```python
from build123d import *

# Parameters (mm, degrees)
SKETCH3_W           = 50.8
SKETCH3_H           = 25.4
SKETCH3_W_2         = 45.72
SKETCH3_H_2         = 20.32
BOSS_EXTRUDE1_DEPTH = 711.2
SKETCH5_R           = 5.08
CUT_EXTRUDE2_DEPTH  = 127


with BuildPart() as part:
    # Sketch3 → Boss-Extrude1 (new body)
    with BuildSketch(Plane(origin=(0, 0, 0), x_dir=(0, 0, -1), z_dir=(1, 0, 0))):
        with Locations((5.321216632, -1.999606833)):
            Rectangle(SKETCH3_W, SKETCH3_H)
        with Locations((5.321216632, -1.999606833)):
            Rectangle(SKETCH3_W_2, SKETCH3_H_2, mode=Mode.SUBTRACT)
    extrude(amount=BOSS_EXTRUDE1_DEPTH)

    # Sketch5 → Cut-Extrude2 (cut)
    with BuildSketch(Plane.XY.offset(20.078783368)):
        with Locations((10.978833808, -1.999606833)):
            Circle(SKETCH5_R)
        with Locations((36.378833808, -1.999606833)):
            Circle(SKETCH5_R)
        with Locations((61.778833808, -1.999606833)):
            Circle(SKETCH5_R)
        with Locations((87.178833808, -1.999606833)):
            Circle(SKETCH5_R)
        with Locations((112.578833808, -1.999606833)):
            Circle(SKETCH5_R)
        with Locations((137.978833808, -1.999606833)):
            Circle(SKETCH5_R)
        with Locations((163.378833808, -1.999606833)):
            Circle(SKETCH5_R)
        with Locations((188.778833808, -1.999606833)):
            Circle(SKETCH5_R)
        with Locations((214.178833808, -1.999606833)):
            Circle(SKETCH5_R)
        with Locations((239.578833808, -1.999606833)):
            Circle(SKETCH5_R)
        with Locations((264.978833808, -1.999606833)):
            Circle(SKETCH5_R)
        with Locations((290.378833808, -1.999606833)):
            Circle(SKETCH5_R)
        with Locations((315.778833808, -1.999606833)):
            Circle(SKETCH5_R)
        with Locations((341.178833808, -1.999606833)):
            Circle(SKETCH5_R)
        with Locations((366.578833808, -1.999606833)):
            Circle(SKETCH5_R)
        with Locations((391.978833808, -1.999606833)):
            Circle(SKETCH5_R)
        with Locations((417.378833808, -1.999606833)):
            Circle(SKETCH5_R)
        with Locations((442.778833808, -1.999606833)):
            Circle(SKETCH5_R)
        with Locations((468.178833808, -1.999606833)):
            Circle(SKETCH5_R)
        with Locations((493.578833808, -1.999606833)):
            Circle(SKETCH5_R)
        with Locations((518.978833808, -1.999606833)):
            Circle(SKETCH5_R)
        with Locations((544.378833808, -1.999606833)):
            Circle(SKETCH5_R)
        with Locations((569.778833808, -1.999606833)):
            Circle(SKETCH5_R)
        with Locations((595.178833808, -1.999606833)):
            Circle(SKETCH5_R)
        with Locations((620.578833808, -1.999606833)):
            Circle(SKETCH5_R)
        with Locations((645.978833808, -1.999606833)):
            Circle(SKETCH5_R)
        with Locations((671.378833808, -1.999606833)):
            Circle(SKETCH5_R)
        with Locations((696.778833808, -1.999606833)):
            Circle(SKETCH5_R)
    extrude(amount=-CUT_EXTRUDE2_DEPTH, mode=Mode.SUBTRACT)


solid = part.part
```
The listing builds one solid part. Answer for the finished solid, in the listing's coordinates (mm). A direction names the side the tool comes from. Give positions to 0.01 mm unless a question says otherwise; leave off trailing zeros. Order: outer loops, then holes, each group sorted by start corner. A loop starts at its lowest first (then second) coordinate and runs counter-clockwise, first axis right, second up.
1) Find section A-A on z = 2.5. Write down the section's boundary in (x, y), then the cut area to 3 significant figures.
Reported:
outline: (0, -14.7) - (711.2, -14.7) - (711.2, -12.16) - (0, -12.16) - close; (0, 8.16) - (711.2, 8.16) - (711.2, 10.7) - (0, 10.7) - close
area: 3,610 mm2
2) Consider line 1 along Z through (x, y) = (43.5, 2.75); line 2 along Y through (x, z) = (214, 4.5); line 3 along Y through (x, z) = (235, -29). Determine where each line is inside the solid, lowest interval first.
Reported:
line 1: z = -30.72 to -28.18, 17.54 to 20.08
line 2: y = -14.7 to -12.16, 8.16 to 10.7
line 3: y = -14.7 to -4.2, 0.2 to 10.7
3) For faces 5 (the face through (351, -14.7, -5)), 6 (the face through (351, 8.16, -5)), determine the directions among +Z, -Z, +X, -X, +Y, -Y from which every point of the face is accessible in a straight line to the end or side of a thin tool.
Reported:
face 5: +Z, -Z, +X, -X, -Y
face 6: +X, -X
4) Determine the mould class of faces 1 (the face through (430, -2, -28.181)), 2 (the face through (351, -12.16, -5)), 3 (the face through (351, -2, 20.079)), 4 (the face through (351, -2, -30.721)) for opening direction Z: pulls with the +Z half, pulls with the -Z half, needs draft (parallel to the pull), parting line crosses it, or undercut.
Reported:
face 1: undercut
face 2: undercut
face 3: pulls with the +Z half
face 4: pulls with the -Z half
